Work out the finished part from the listing and answer in its coordinate system (mm). Face numbers are marked on the shaded views. A direction names the side the tool comes from. Give positions to 0.01 mm unless a question says otherwise; leave off trailing zeros. Order: outer loops, then holes, each group sorted by start corner. A loop starts at its lowest first (then second) coordinate and runs counter-clockwise, first axis right, second up.
```python
from build123d import *

# Parameters (mm, degrees)
BOSS_EXTRUDE1_DEPTH = 36
CUT_EXTRUDE1_REACH  = 48
SKETCH2_R           = 2.25
CUT_EXTRUDE2_REACH  = 8
SKETCH3_R           = 2.25
SKETCH4_R           = 4
CUT_EXTRUDE3_DEPTH  = 4
SKETCH5_R           = 4
CUT_EXTRUDE4_DEPTH  = 4
CUT_EXTRUDE5_REACH  = 48
SKETCH7_R           = 2.25
SKETCH8_R           = 2.75
CUT_EXTRUDE6_DEPTH  = 4
BOSS_EXTRUDE2_DEPTH = 3


with BuildPart() as part:
    # Sketch1 → Boss-Extrude1 (new body, symmetric)
    with BuildSketch(Plane(origin=(0, 0, 0), x_dir=(0, 0, -1), z_dir=(1, 0, 0))):
        Polygon((-20, 20), (20, 20), (20, -20), (26, -20), (26, 20), (60, 20), (60, 26), (-20, 26), align=None)
    extrude(amount=BOSS_EXTRUDE1_DEPTH, both=True)

    # Sketch2 → Cut-Extrude1 (cut, up to next)
    with BuildSketch(Plane(origin=(0, 0, -26), x_dir=(-1, 0, 0), z_dir=(0, 0, -1)), mode=Mode.PRIVATE) as cut_extrude1_sk1:
        with Locations((-22.5, 0)):
            Circle(SKETCH2_R)
    cut_extrude1_tool1 = extrude(cut_extrude1_sk1.sketch, amount=-CUT_EXTRUDE1_REACH, mode=Mode.PRIVATE) & part.part
    add(cut_extrude1_tool1.solids().sort_by_distance((22.5, 0, -26))[0], mode=Mode.SUBTRACT)
    # Sketch2 → Cut-Extrude1 (cut, up to next)
    with BuildSketch(Plane(origin=(0, 0, -26), x_dir=(-1, 0, 0), z_dir=(0, 0, -1)), mode=Mode.PRIVATE) as cut_extrude1_sk2:
        with Locations((22.5, 0)):
            Circle(SKETCH2_R)
    cut_extrude1_tool2 = extrude(cut_extrude1_sk2.sketch, amount=-CUT_EXTRUDE1_REACH, mode=Mode.PRIVATE) & part.part
    add(cut_extrude1_tool2.solids().sort_by_distance((-22.5, 0, -26))[0], mode=Mode.SUBTRACT)

    # Sketch3 → Cut-Extrude2 (cut, up to next)
    with BuildSketch(Plane.XZ.offset(-20), mode=Mode.PRIVATE) as cut_extrude2_sk1:
        Circle(SKETCH3_R)
    cut_extrude2_tool1 = extrude(cut_extrude2_sk1.sketch, amount=-CUT_EXTRUDE2_REACH, mode=Mode.PRIVATE) & part.part
    add(cut_extrude2_tool1.solids().sort_by_distance((0, 20, 0))[0], mode=Mode.SUBTRACT)

    # Sketch4 → Cut-Extrude3 (cut)
    with BuildSketch(Plane(origin=(0, 0, -26), x_dir=(-1, 0, 0), z_dir=(0, 0, -1))):
        with Locations((-22.5, 0)):
            Circle(SKETCH4_R)
        with Locations((22.5, 0)):
            Circle(SKETCH4_R)
    extrude(amount=-CUT_EXTRUDE3_DEPTH, mode=Mode.SUBTRACT)

    # Sketch5 → Cut-Extrude4 (cut)
    with BuildSketch(Plane(origin=(0, 26, 0), x_dir=(1, 0, 0), z_dir=(0, 1, 0))):
        Circle(SKETCH5_R)
    extrude(amount=-CUT_EXTRUDE4_DEPTH, mode=Mode.SUBTRACT)

    # Sketch7 → Cut-Extrude5 (cut, up to next)
    with BuildSketch(Plane(origin=(0, 26, 0), x_dir=(1, 0, 0), z_dir=(0, 1, 0)), mode=Mode.PRIVATE) as cut_extrude5_sk1:
        with Locations((-22.375, 8.95)):
            Circle(SKETCH7_R)
    cut_extrude5_tool1 = extrude(cut_extrude5_sk1.sketch, amount=-CUT_EXTRUDE5_REACH, mode=Mode.PRIVATE) & part.part
    add(cut_extrude5_tool1.solids().sort_by_distance((-22.375, 26, -8.95))[0], mode=Mode.SUBTRACT)
    # Sketch7 → Cut-Extrude5 (cut, up to next)
    with BuildSketch(Plane(origin=(0, 26, 0), x_dir=(1, 0, 0), z_dir=(0, 1, 0)), mode=Mode.PRIVATE) as cut_extrude5_sk2:
        with Locations((22.375, 8.95)):
            Circle(SKETCH7_R)
    cut_extrude5_tool2 = extrude(cut_extrude5_sk2.sketch, amount=-CUT_EXTRUDE5_REACH, mode=Mode.PRIVATE) & part.part
    add(cut_extrude5_tool2.solids().sort_by_distance((22.375, 26, -8.95))[0], mode=Mode.SUBTRACT)

    # Sketch8 → Cut-Extrude6 (cut)
    with BuildSketch(Plane(origin=(0, 26, 0), x_dir=(1, 0, 0), z_dir=(0, 1, 0))):
        with Locations((-22.375, 8.95)):
            Circle(SKETCH8_R)
        with Locations((22.375, 8.95)):
            Circle(SKETCH8_R)
    extrude(amount=-CUT_EXTRUDE6_DEPTH, mode=Mode.SUBTRACT)

    # Sketch9 → Boss-Extrude2 (add, symmetric)
    with BuildSketch(Plane(origin=(0, 0, 0), x_dir=(0, 0, -1), z_dir=(1, 0, 0))):
        Polygon((26, -20), (60, 20), (26, 20), align=None)
    extrude(amount=BOSS_EXTRUDE2_DEPTH, both=True)


solid = part.part
```
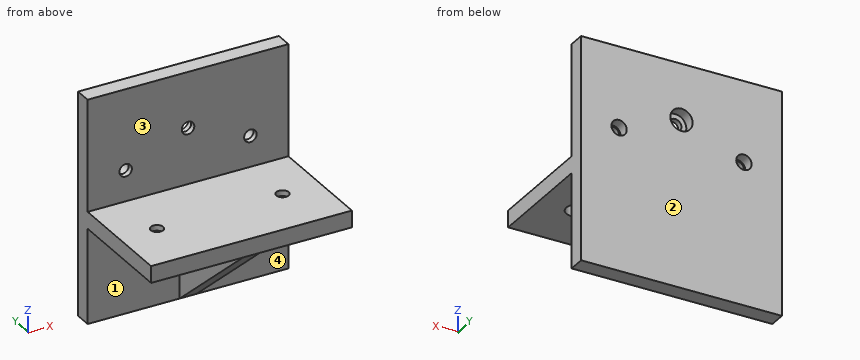
1. Given P1, Ø1, axis at x = 12, z = -35.5, coming from the -Y side; P2, Ø5, axis at x = -22.375, z = -8.95, coming from the +Y side; P3, Ø16.5, axis at x = -22, y = -10, coming from the -Z side; P4, Ø3.5, axis at x = 22.5, y = 0, coming from the -Z side, each flat-ended and moving along its own axis, determine where each tip first touches the part or whether it passes through.
Findings below:
P1: stops at y = 20
P2: stops at y = 22
P3: stops at z = -26
P4: passes through
2. Which of the six approach directions +Z, -Z, +X, -X, +Y, -Y give full straight-line access (tool end or side, diameter ignored) to the marked faces 1, 2, 3 and 4?
Findings below:
face 1: -Z, -X, -Y
face 2: +Z, -Z, +X, -X, +Y
face 3: +Z, +X, -X, -Y
face 4: -Z, +X, -Y
3. Straight lines are drawn through the part: probe 1 along X at (y, z) = (21.2, -8.95) (3 decimals); probe 2 along X at (y, z) = (23, -7); probe 3 along Y at (x, z) = (22.5, -25.1). For each, find the intervals that lie inside material, in ascending order.
Findings below:
probe 1: x = -36 to -24.625, -20.125 to 20.125, 24.625 to 36
probe 2: x = -36 to -24.31, -20.44 to 20.44, 24.31 to 36
probe 3: y = -20 to -4, 4 to 26
4. The part is cut by section A-A (z = -8.95). Write down the section's boundary in (x, y) (3 decimals), then the cut area to 3 significant figures.
Findings below:
outline: (-36, 20) - (-24.625, 20) - (-24.625, 22) - (-25.125, 22) - (-25.125, 26) - (-36, 26) - close; (-20.125, 20) - (20.125, 20) - (20.125, 22) - (19.625, 22) - (19.625, 26) - (-19.625, 26) - (-19.625, 22) - (-20.125, 22) - close; (24.625, 20) - (36, 20) - (36, 26) - (25.125, 26) - (25.125, 22) - (24.625, 22) - close
area: 370 mm2
5. The part is cut by section B-B (y = 0). Write down the section's boundary in (x, z).
Findings below:
outline: (-36, -26) - (-26.5, -26) - (-26.5, -22) - (-24.75, -22) - (-24.75, -20) - (-36, -20) - close; (-20.25, -22) - (-18.5, -22) - (-18.5, -26) - (-3, -26) - (-3, -43) - (3, -43) - (3, -26) - (18.5, -26) - (18.5, -22) - (20.25, -22) - (20.25, -20) - (-20.25, -20) - close; (24.75, -22) - (26.5, -22) - (26.5, -26) - (36, -26) - (36, -20) - (24.75, -20) - close
6. The part is cut by section C-C (z = 0). Write down the section's boundary in (x, y).
Findings below:
outline: (-36, 20) - (-2.25, 20) - (-2.25, 22) - (-4, 22) - (-4, 26) - (-36, 26) - close; (2.25, 20) - (36, 20) - (36, 26) - (4, 26) - (4, 22) - (2.25, 22) - close
7. The part is cut by section D-D (x = 0). Write down the section's boundary in (y, z), then the cut area to 3 significant figures.
Findings below:
outline: (-20, -26) - (20, -60) - (26, -60) - (26, -4) - (22, -4) - (22, -2.25) - (20, -2.25) - (20, -20) - (-20, -20) - close; (20, 2.25) - (22, 2.25) - (22, 4) - (26, 4) - (26, 20) - (20, 20) - close
area: 1,360 mm2
